```python
from build123d import *

# Parameters (mm, degrees)
F1_DEPTH = 76.2
F2_W     = 30.3190927953
F2_H     = 20.7057222724
F4_DEPTH = 2.794


# Not quite as in the source:
# - the program builds the solid bodies; features that only make, move or delete a surface that nothing else refers to are left out


with BuildPart() as f1:
    # F0 (on Front) → F1 (new body)
    with BuildSketch(Plane.XZ):
        Polygon((-93.7673449516, 21.5931143612), (-93.7673449516, 21.2973169982), (-93.7673449516, 12.9849165678), (-76.1796534061, -2.6621618308), (-63.4482521564, -2.6621618308), (-63.4482521564, 21.4452156797), align=None)
        Polygon((-63.4482521564, 42.0030392706), (-63.4482521564, 21.4452156797), (-33.1291593611, 21.2973169982), (-33.1291593611, 42.0030392706), align=None)
        Polygon((-93.7673449516, 42.0030392706), (-93.7673449516, 21.5931143612), (-63.4482521564, 21.4452156797), (-63.4482521564, 42.0030392706), align=None)
        with BuildLine():
            Line((30.7627860457, 21.2973169982), (-33.1291593611, 21.2973169982))
            Line((-33.1291593611, 21.2973169982), (-47.1545420587, -2.6621618308))
            Line((-47.1545420587, -2.6621618308), (-16.8603751808, -2.6621618308))
            ThreePointArc((-16.8603751808, -2.6621618308), (-4.7327380162, 7.2386136425), (7.3948991485, -2.6621618308))
            Line((7.3948991485, -2.6621618308), (30.7627860457, -2.6621618308))
            Line((30.7627860457, -2.6621618308), (30.7627860457, 21.2973169982))
        make_face()
        with BuildLine():
            Line((-93.7673449516, 21.2973169982), (-128.96707654, 21.2973169982))
            Line((-128.96707654, 21.2973169982), (-129.2628794909, -2.6621618308))
            Line((-129.2628794909, -2.6621618308), (-104.1202098131, -2.6621618308))
            ThreePointArc((-104.1202098131, -2.6621618308), (-92.8799584508, 6.8226352019), (-81.6397070885, -2.6621618308))
            Line((-81.6397070885, -2.6621618308), (-76.1796534061, -2.6621618308))
            Line((-76.1796534061, -2.6621618308), (-93.7673449516, 12.9849165678))
            Line((-93.7673449516, 12.9849165678), (-93.7673449516, 21.2973169982))
        make_face()
        Polygon((-33.1291593611, 21.2973169982), (-63.4482521564, 21.4452156797), (-63.4482521564, -2.6621618308), (-47.1545420587, -2.6621618308), align=None)
    extrude(amount=F1_DEPTH)

    # F2 (on face) → F4 (join)
    with BuildSketch(Plane.XZ.offset(76.2)):
        with Locations((-78.607798554, 31.6501781344)):
            Rectangle(F2_W, F2_H)
        Polygon((-90.9339487553, 39.8703143001), (-65.8644288778, 39.8703143001), (-66.4106756449, 23.5412772745), (-90.9339487553, 23.5412772745), align=None, mode=Mode.SUBTRACT)
        with Locations((-48.2887057588, 31.6501781344)):
            Rectangle(F2_W, F2_H)
        Polygon((-35.3044308722, 23.5412772745), (-61.6788230836, 23.5412772745), (-61.5411959589, 39.8703143001), (-35.3044308722, 39.8703143001), align=None, mode=Mode.SUBTRACT)
        Polygon((-63.4482521564, 21.2973169982), (-93.7673449516, 21.2973169982), (-75.8718252182, -2.6621618308), (-63.4482521564, -2.6621618308), align=None)
        Polygon((-33.1291593611, 21.2973169982), (-63.4482521564, 21.2973169982), (-63.4482521564, -2.6621618308), (-49.2500411347, -2.6621618308), align=None)
        Polygon((-57.2931170464, 16.1802023649), (-61.0887669027, 16.1802023649), (-61.2885393202, 19.1765353084), (-57.2931170464, 19.1765353084), align=None, mode=Mode.SUBTRACT)
    extrude(amount=F4_DEPTH)


solid = f1.part
```
Geometry: final body of the model. Coordinates: model frame, mm. A direction names the side the tool comes from. Round coordinates to 2 decimals unless told otherwise and drop trailing zeros. Write each loop counter-clockwise with the first axis right and the second up, starting at its lowest first coordinate (ties: lowest second). Pieces come first, ordered by that corner, then holes. Notation, with made-up numbers: (66.25, 22) -> (95.25, 22) arc R17 cw to (95.25, 41) -> close; hole circle Ø7 at (-31, 24). An arc over 180 degrees is marked (long way). Return JSON: item names as keys, results as strings.
Q1. Section D-D on x = -87.5. Return the cut outline in (y, z), and give its area (3 significant figures).
From the geometry:
{"outline": "(-78.99, 12.91) -> (-76.2, 12.91) -> (-76.2, 5.47) -> (0, 5.47) -> (0, 42) -> (-78.99, 42) -> (-78.99, 39.87) -> (-76.2, 39.87) -> (-76.2, 23.54) -> (-78.99, 23.54) -> close", "area": "2,820 mm2"}
Q2. Section A-A on y = -74. Return the cut outline in (x, z).
From the geometry:
{"outline": "(-129.26, -2.66) -> (-104.12, -2.66) arc R11.4 cw to (-81.64, -2.66) -> (-16.86, -2.66) arc R12.38 cw to (7.39, -2.66) -> (30.76, -2.66) -> (30.76, 21.3) -> (-33.13, 21.3) -> (-33.13, 42) -> (-93.77, 42) -> (-93.77, 21.3) -> (-128.97, 21.3) -> close"}
Q3. Mould query, pull axis Z, two halves, no side actions, for faces 1 (the cylindrical face through (-93.1, -37.57, 6.82)), 2 (the flat face through (-109, -76.2, 9)), 3 (the flat face through (-49, -76.2, 32)). Classes: +Z half, -Z half, draft (parallel to the pull), parting line (faces both ways), or undercut.
From the geometry:
{"face 1": "-Z half", "face 2": "draft", "face 3": "undercut"}
Q4. Section C-C on x = -116. Return the cut outline in (y, z).
From the geometry:
{"outline": "(-76.2, -2.66) -> (0, -2.66) -> (0, 21.3) -> (-76.2, 21.3) -> close"}
Q5. Section B-B on z = 33. Return the cut outline in (x, y).
From the geometry:
{"outline": "(-93.77, -78.99) -> (-90.93, -78.99) -> (-90.93, -76.2) -> (-66.09, -76.2) -> (-66.09, -78.99) -> (-61.6, -78.99) -> (-61.6, -76.2) -> (-35.3, -76.2) -> (-35.3, -78.99) -> (-33.13, -78.99) -> (-33.13, 0) -> (-93.77, 0) -> close"}
Q6. First-contact query: pin 1 Ø6 at (y, z) = (-46.5, 31) entering from +X; pin 2 Ø8 at (x, z) = (-15, 26) entering from +Y; pin 3 Ø8 at (x, y) = (-93.5, -60.5) entering from -Z; pin 4 Ø12 at (x, z) = (9, 13) entering from -Y. Flat tips, straight axial feed; report the tip coordinate or a pass-through.
From the geometry:
{"pin 1": "x = -33.13", "pin 2": "through", "pin 3": "z = 5.84", "pin 4": "y = -76.2"}
Q7. Set-up query: faces 4 (the flat face through (-93.767, -39, 32)), 5 (the flat face through (-1, -38, 21.297)), 6 (the flat face through (-35.304, -78, 32)). Return all of +Z, -Z, +X, -X, +Y, -Y with unobstructed straight access to the full face (end or side cutting, diameter ignored); none if empty.
From the geometry:
{"face 4": "+Z, -X, +Y, -Y", "face 5": "+Z, +X, +Y, -Y", "face 6": "-Y"}
Q8. Ray query, line 1 (X direction, y = -43, z = 4.5); line 2 (X direction, y = -9, z = 5.5); line 3 (Y direction, x = -32, z = 19.5). Return the intervals inside material, ascending.
From the geometry:
{"line 1": "-129.17 to -99.78, -85.98 to -12.5, 3.03 to 30.76", "line 2": "-129.16 to -98.21, -87.55 to -11.06, 1.59 to 30.76", "line 3": "-76.2 to 0"}
